Answer from the drawing. Dimensions are ordinates in mm from the lowest x, y and z of the part. A direction names the side the tool comes from. Give positions to 0.01 mm unless a question says otherwise; leave off trailing zeros. Loops run counter-clockwise (first coordinate to the right, second up) from the corner with the lowest first, then second, coordinate; pieces in that order, holes last.
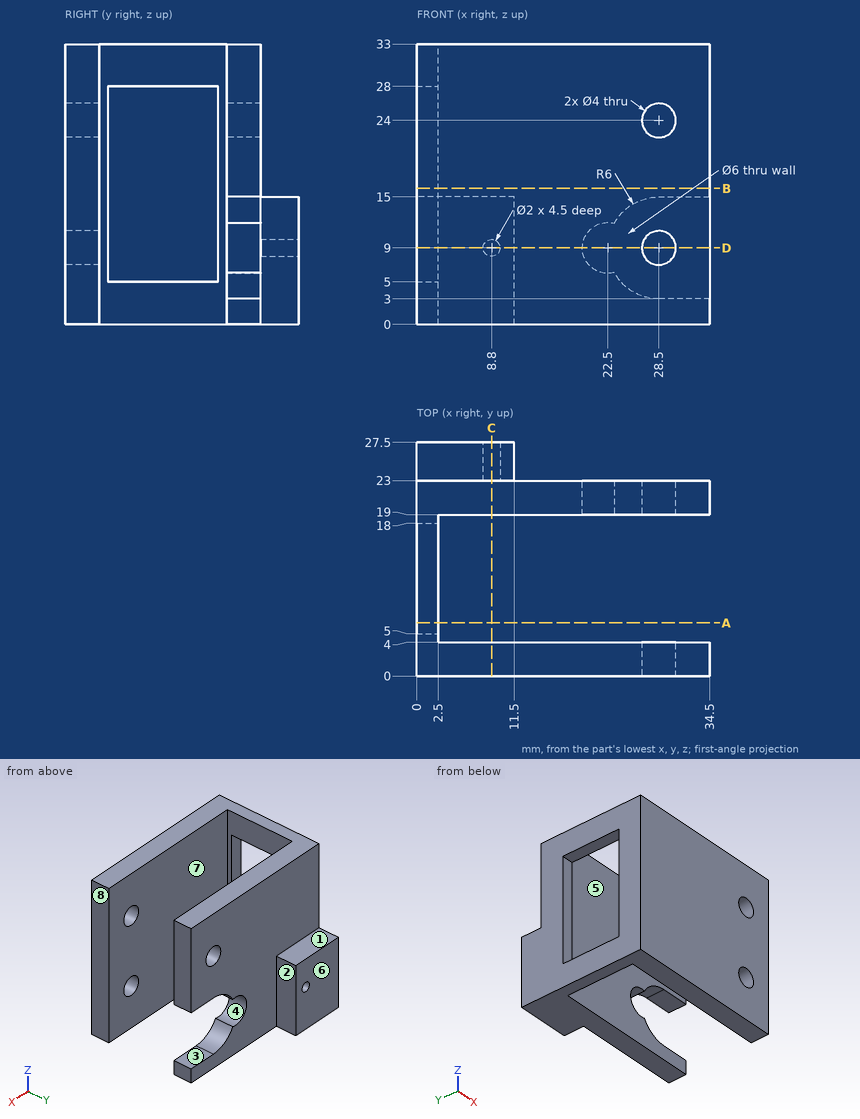
Item 1: Determine the mould class of the marked faces 5, 6, 7 and 8 for opening direction Y: released by +Y, released by -Y, zero draft, split by the parting line, or undercut.
Item 2: A flat-ended cylindrical pin translates along its axis: pin 1 Ø4 at (x, z) = (23.5, 23) entering from +Y. Find the tip coordinate at first contact, or state that the pin passes through.
Item 3: Consider line 1 (Z direction, x = 28.5, y = 2.35); line 2 (Y direction, x = 6, z = 21); line 3 (Z direction, x = 8.8, y = 24.05). Determine where each line is inside the solid, lowest interval first.
Item 4: Find section D-D, the plane z = 9. Write down the section's boundary in (x, y).
Item 5: Find section A-A, the plane y = 6.25. Write down the section's boundary in (x, z), plus the area to 3 significant figures.
Item 6: Find section C-C, the plane x = 8.8. Write down the section's boundary in (y, z), plus the area to 4 significant figures.
Item 7: Find section B-B, the plane z = 16. Write down the section's boundary in (x, y), plus the area to 3 significant figures.
Item 8: For the marked faces 1, 2, 3 and 4, determine the directions among +Z, -Z, +X, -X, +Y, -Y from which every point of the face is accessible in a straight line to the end or side of a thin tool.
Ans:
1. face 5: undercut
1. face 6: released by +Y
1. face 7: undercut
1. face 8: zero draft
2. pin 1: stops at y = 23
3. line 1: z = 0 to 7, 11 to 22, 26 to 33
3. line 2: y = 0 to 4, 19 to 23
3. line 3: z = 0 to 8, 10 to 15
4. outline: (0, 0) - (26.5, 0) - (26.5, 4) - (2.5, 4) - (2.5, 5) - (0, 5) - close; (0, 18) - (2.5, 18) - (2.5, 19) - (19.5, 19) - (19.5, 23) - (11.5, 23) - (11.5, 27.5) - (9.8, 27.5) - (9.8, 23) - (7.8, 23) - (7.8, 27.5) - (0, 27.5) - close; (30.5, 0) - (34.5, 0) - (34.5, 4) - (30.5, 4) - close
5. outline: (0, 0) - (2.5, 0) - (2.5, 5) - (0, 5) - close; (0, 28) - (2.5, 28) - (2.5, 33) - (0, 33) - close
5. area: 25.0 mm2
6. outline: (0, 0) - (4, 0) - (4, 33) - (0, 33) - close; (19, 0) - (27.5, 0) - (27.5, 8) - (23, 8) - (23, 10) - (27.5, 10) - (27.5, 15) - (23, 15) - (23, 33) - (19, 33) - close
6. area: 322.5 mm2
7. outline: (0, 0) - (34.5, 0) - (34.5, 4) - (2.5, 4) - (2.5, 5) - (0, 5) - close; (0, 18) - (2.5, 18) - (2.5, 19) - (34.5, 19) - (34.5, 23) - (0, 23) - close
7. area: 281 mm2
8. face 1: +Z, +X, -X, +Y
8. face 2: +Z, -Z, +X, +Y
8. face 3: +X, +Y
8. face 4: +Y
